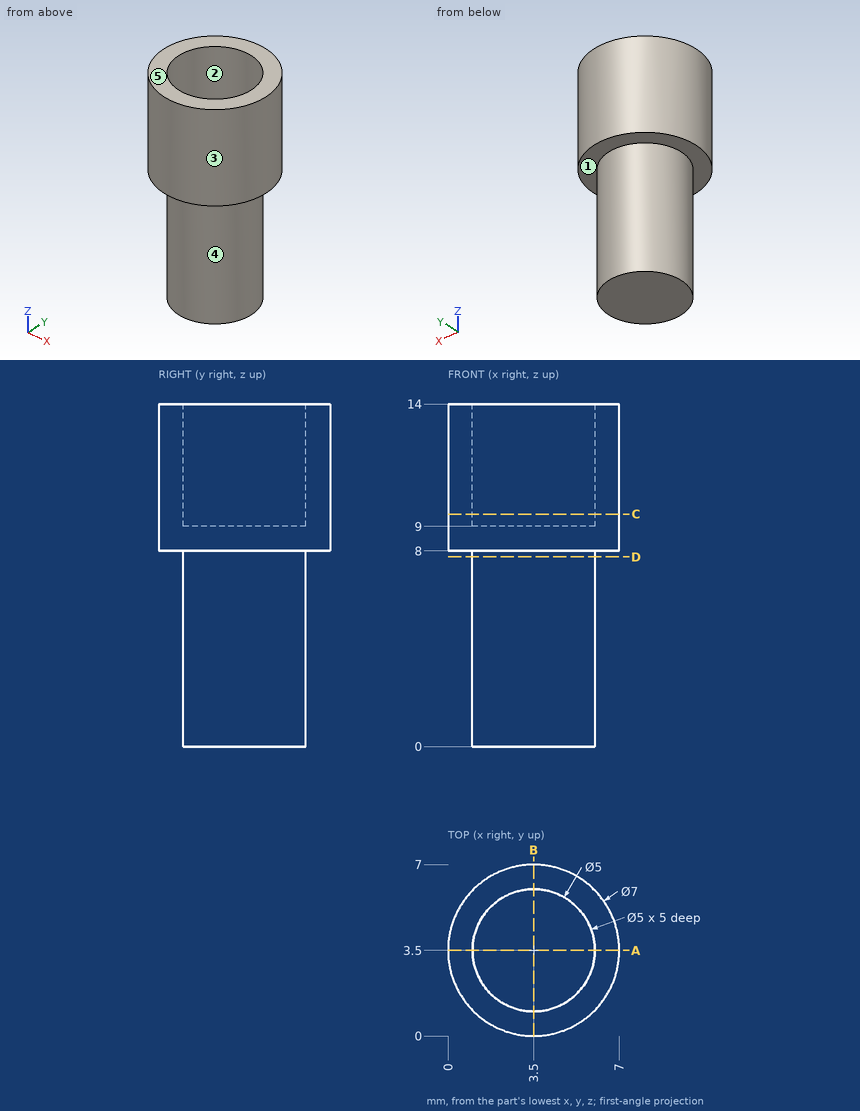
Verification items for this drawing (mm, ordinates from the low corner). A direction names the side the tool comes from. Coordinates: 2 decimals unless noted, no trailing zeros. Order: outer loops, then holes, each group sorted by start corner. A loop starts at its lowest first (then second) coordinate and runs counter-clockwise, first axis right, second up. Notation, with made-up numbers: (31.25, -32) - (68.25, -32) arc R9 ccw to (68.25, -28) - close; hole circle Ø5 at (0, -12.5). An arc over 180 degrees is marked (long way). Answer as a JSON object with one key per item and string values. Group by question number.
Item 1: Tool access check on the marked faces 4 and 5. Record the directions out of +Z, -Z, +X, -X, +Y, -Y that give a thin tool (end or side, any length) a straight path to the whole face; none if there is none.
Item 2: Draft check along Y on the marked faces 1, 2 and 3. Enter one of: +Y half, -Y half, draft (parallel to the pull), parting line (faces both ways), or undercut.
Item 3: Sectioned sample at C-C, the plane z = 9.5. Record the cut outline in (x, y), and give its area (3 significant figures).
Item 4: Depth check by flat-ended pin: pin 1 Ø3 at (x, z) = (4.5, 9) entering from -Y; pin 2 Ø1 at (x, y) = (0.5, 4) entering from -Z; pin 3 Ø3 at (x, z) = (6, 4) entering from -Y; pin 4 Ø2 at (x, z) = (4.5, 3) entering from -Y. Enter the tip coordinate at first touch or a pass-through.
Item 5: Scan lines: probe 1 along Y at (x, z) = (3.5, 12.75); probe 2 along Z at (x, y) = (3, 6.75); probe 3 along Z at (x, y) = (2.5, 3.25). Record each from-to range of solid material in increasing order.
Item 6: Sectioned sample at D-D, the plane z = 7.75. Record the cut outline in (x, y), and give its area (3 significant figures).
Item 7: Sectioned sample at A-A, the plane y = 3.5. Record the cut outline in (x, z).
Resolved:
{
 "1": {"face 4": "-Z", "face 5": "+Z, +X, -X, +Y, -Y"},
 "2": {"face 1": "draft", "face 2": "undercut", "face 3": "parting line"},
 "3": {"outline": "circle Ø7 at (3.5, 3.5); hole circle Ø5 at (3.5, 3.5)", "area": "18.8 mm^2"},
 "4": {"pin 1": "y = 0", "pin 2": "z = 8", "pin 3": "y = 1.21", "pin 4": "y = 1"},
 "5": {"probe 1": "0 to 1, 6 to 7", "probe 2": "8 to 14", "probe 3": "0 to 9"},
 "6": {"outline": "circle Ø5 at (3.5, 3.5)", "area": "19.6 mm^2"},
 "7": {"outline": "(0, 8) - (1, 8) - (1, 0) - (6, 0) - (6, 8) - (7, 8) - (7, 14) - (6, 14) - (6, 9) - (1, 9) - (1, 14) - (0, 14) - close"}
}
